Part model, mm, in its own coordinate system. Face numbers are marked on the shaded views. Give positions to 0.01 mm unless a question says otherwise; leave off trailing zeros. Loops run counter-clockwise (first coordinate to the right, second up) from the corner with the lowest first, then second, coordinate; pieces in that order, holes last. Notation, with made-up numbers: (74, 13) -> (133, 13) arc R21 cw to (133, 21) -> close; hole circle Ø2 at (46.5, -21). An arc over 180 degrees is marked (long way). One line per question, with ' | ' between items.
Autodesk Inventor part; units mm, degrees
ref_plane "Work Plane4" through (0, 0, -44.52672) normal (1, 0, 0) x (0, 0.9903099, -0.1388753)
ref_plane "YZ Plane" through (0, 0, 0) normal (1, 0, 0) x (0, 1, 0)
ref_plane "XZ Plane" through (0, 0, 0) normal (0, 1, 0) x (-1, 0, 0)
sketch "Sketch1" plane through (0, 0, 0) normal (0, 1, 0) x (-1, 0, 0)
  circle A0 centre (0, 0) radius 110 construction
  arc A1 (43.0581, -98.5) -> (-43.0581, -98.5) centre (0, 0) ccw
  line L0 (0, -107.5) -> (0, -98.5) construction
  line L1 (0, -98.5) -> (0, -73.5) construction
  line L2 (0, -98.5) -> (-43.0581, -98.5) construction
  line L3 (0, -98.5) -> (43.0581, -98.5) construction
  line L4 (43.0581, -98.5) -> (-43.0581, -98.5) construction
  line L5 (-18.0581, -73.5) -> (18.0581, -73.5)
  arc A2 (43.0581, -98.5) -> (18.0581, -73.5) centre (18.0581, -98.5) ccw
  arc A3 (-18.0581, -73.5) -> (-43.0581, -98.5) centre (-18.0581, -98.5) ccw
  line L6 (0, 107.5) -> (0, 97.5) construction
  line L7 (0, 97.5) -> (-22.5, 97.5) construction
  line L8 (-22.5, 97.5) -> (-22.5, 82.5) construction
  line L9 (22.5, 82.5) -> (22.5, 97.5) construction
  line L10 (22.5, 90) -> (-22.5, 90) construction
  line L11 (15, 97.5) -> (-15, 97.5)
  line L12 (-15, 82.5) -> (15, 82.5)
  arc A4 (15, 82.5) -> (15, 97.5) centre (15, 90) ccw
  arc A5 (-15, 97.5) -> (-15, 82.5) centre (-15, 90) ccw
  line L13 (22.5, 82.5) -> (17.5, 82.5) construction
  line L14 (17.5, 82.5) -> (17.5, 77.5) construction
  circle A6 centre (17.5, 77.5) radius 1.6
  circle A7 centre (-17.5, 77.5) radius 1.6
  line L15 (-58.336309, 79.549513) -> (-79.549513, 58.336309)
  arc A8 (-47.729708, 68.942911) -> (-58.336309, 79.549513) centre (-53.033009, 74.246212) ccw
  arc A9 (-79.549513, 58.336309) -> (-68.942911, 47.729708) centre (-74.246212, 53.033009) ccw
  line L16 (-68.942911, 47.729708) -> (-47.729708, 68.942911)
  circle A10 centre (-67.175144, 42.426407) radius 1.6
  circle A11 centre (-42.426407, 67.175144) radius 1.6
  line L17 (-97.5, 15) -> (-97.5, -15)
  arc A12 (-82.5, 15) -> (-97.5, 15) centre (-90, 15) ccw
  arc A13 (-97.5, -15) -> (-82.5, -15) centre (-90, -15) ccw
  line L18 (-82.5, -15) -> (-82.5, 15)
  circle A14 centre (-77.5, -17.5) radius 1.6
  circle A15 centre (-77.5, 17.5) radius 1.6
  line L19 (-79.549513, -58.336309) -> (-58.336309, -79.549513)
  arc A16 (-68.942911, -47.729708) -> (-79.549513, -58.336309) centre (-74.246212, -53.033009) ccw
  arc A17 (-58.336309, -79.549513) -> (-47.729708, -68.942911) centre (-53.033009, -74.246212) ccw
  line L20 (-47.729708, -68.942911) -> (-68.942911, -47.729708)
  circle A18 centre (-42.426407, -67.175144) radius 1.6
  circle A19 centre (-67.175144, -42.426407) radius 1.6
  line L21 (-15, -97.5) -> (15, -97.5)
  arc A20 (-15, -82.5) -> (-15, -97.5) centre (-15, -90) ccw
  arc A21 (15, -97.5) -> (15, -82.5) centre (15, -90) ccw
  line L22 (15, -82.5) -> (-15, -82.5)
  circle A22 centre (17.5, -77.5) radius 1.6
  circle A23 centre (-17.5, -77.5) radius 1.6
  line L23 (58.336309, -79.549513) -> (79.549513, -58.336309)
  arc A24 (47.729708, -68.942911) -> (58.336309, -79.549513) centre (53.033009, -74.246212) ccw
  arc A25 (79.549513, -58.336309) -> (68.942911, -47.729708) centre (74.246212, -53.033009) ccw
  line L24 (68.942911, -47.729708) -> (47.729708, -68.942911)
  circle A26 centre (67.175144, -42.426407) radius 1.6
  circle A27 centre (42.426407, -67.175144) radius 1.6
  line L25 (97.5, -15) -> (97.5, 15)
  arc A28 (82.5, -15) -> (97.5, -15) centre (90, -15) ccw
  arc A29 (97.5, 15) -> (82.5, 15) centre (90, 15) ccw
  line L26 (82.5, 15) -> (82.5, -15)
  circle A30 centre (77.5, 17.5) radius 1.6
  circle A31 centre (77.5, -17.5) radius 1.6
  line L27 (79.549513, 58.336309) -> (58.336309, 79.549513)
  arc A32 (68.942911, 47.729708) -> (79.549513, 58.336309) centre (74.246212, 53.033009) ccw
  arc A33 (58.336309, 79.549513) -> (47.729708, 68.942911) centre (53.033009, 74.246212) ccw
  line L28 (47.729708, 68.942911) -> (68.942911, 47.729708)
  circle A34 centre (42.426407, 67.175144) radius 1.6
  circle A35 centre (67.175144, 42.426407) radius 1.6
  line L29 (58.336309, -58.336309) -> (51.265242, -51.265242) construction
  line L30 (40.65864, -61.871843) -> (61.871843, -40.65864)
  arc A36 (40.65864, -61.871843) -> (44.52672, -89.539774) centre (53.033009, -74.246212) ccw
  arc A37 (89.539774, -44.52672) -> (61.871843, -40.65864) centre (74.246212, -53.033009) ccw
  line L31 (0, -73.5) -> (0, -66.5) construction
  arc A38 (44.52672, 89.539774) -> (40.65864, 61.871843) centre (53.033009, 74.246212) ccw
  line L32 (61.871843, 40.65864) -> (40.65864, 61.871843)
  arc A39 (61.871843, 40.65864) -> (89.539774, 44.52672) centre (74.246212, 53.033009) ccw
  arc A40 (-89.539774, 44.52672) -> (-61.871843, 40.65864) centre (-74.246212, 53.033009) ccw
  line L33 (-40.65864, 61.871843) -> (-61.871843, 40.65864)
  arc A41 (-40.65864, 61.871843) -> (-44.52672, 89.539774) centre (-53.033009, 74.246212) ccw
  arc A42 (-44.52672, -89.539774) -> (-40.65864, -61.871843) centre (-53.033009, -74.246212) ccw
  line L34 (-61.871843, -40.65864) -> (-40.65864, -61.871843)
  arc A43 (-61.871843, -40.65864) -> (-89.539774, -44.52672) centre (-74.246212, -53.033009) ccw
  arc A44 (89.539774, -44.52672) -> (89.539774, 44.52672) centre (0, 0) ccw
  arc A45 (44.52672, 89.539774) -> (-44.52672, 89.539774) centre (0, 0) ccw
  arc A46 (-89.539774, 44.52672) -> (-89.539774, -44.52672) centre (0, 0) ccw
  line L35 (43.0581, -98.5) -> (48.0581, -98.5) construction
  line L36 (48.0581, -98.5) -> (48.0581, -88.5) construction
  circle A47 centre (48.0581, -88.5) radius 1.6
  circle A48 centre (-48.0581, -88.5) radius 1.6
  line L37 (18.0581, -66.5) -> (-18.0581, -66.5)
  arc A49 (17.5, -66.5) -> (43.0581, -59.472383) centre (19.514525, -23.837671) ccw
  arc A50 (-44.52672, -58.003763) -> (-18.0581, -66.5) centre (-19.508856, -25.542168) ccw
  arc A51 (-48.0581, -88.5) -> (-42.426407, -67.175144) centre (-60.43967, -73.824078) ccw construction
  arc A52 (-48.0581, -88.5) -> (-42.426407, -67.175144) centre (-60.43967, -73.824078) ccw construction
  arc A53 (-44.936716, -92.199789) -> (-37.885276, -65.498953) centre (-60.43967, -73.824078) ccw
  arc A54 (-51.179485, -84.800211) -> (-46.967537, -68.851335) centre (-60.43967, -73.824078) ccw
  arc A55 (-51.179485, -84.800211) -> (-44.936716, -92.199789) centre (-48.0581, -88.5) ccw
  arc A56 (-37.885276, -65.498953) -> (-46.967537, -68.851335) centre (-42.426407, -67.175144) ccw
  line L38 (42.426407, 67.175144) -> (67.175144, 42.426407) construction
  line L39 (45.961941, 70.710678) -> (70.710678, 45.961941)
  line L40 (63.63961, 38.890873) -> (38.890873, 63.63961)
  arc A57 (45.961941, 70.710678) -> (38.890873, 63.63961) centre (42.426407, 67.175144) ccw
  arc A58 (63.63961, 38.890873) -> (70.710678, 45.961941) centre (67.175144, 42.426407) ccw
  line L41 (-42.426407, 67.175144) -> (-67.175144, 42.426407) construction
  line L42 (-45.961941, 70.710678) -> (-70.710678, 45.961941)
  line L43 (-63.63961, 38.890873) -> (-38.890873, 63.63961)
  arc A59 (-38.890873, 63.63961) -> (-45.961941, 70.710678) centre (-42.426407, 67.175144) ccw
  arc A60 (-70.710678, 45.961941) -> (-63.63961, 38.890873) centre (-67.175144, 42.426407) ccw
  line L44 (-42.426407, 67.175144) -> (42.426407, 67.175144) construction
  line L45 (-42.426407, 62.175144) -> (42.426407, 62.175144)
  line L46 (42.426407, 72.175144) -> (-42.426407, 72.175144)
  arc A61 (-42.426407, 72.175144) -> (-42.426407, 62.175144) centre (-42.426407, 67.175144) ccw
  arc A62 (42.426407, 62.175144) -> (42.426407, 72.175144) centre (42.426407, 67.175144) ccw
  line L47 (37.025198, 67.175144) -> (33.025198, 67.175144) construction
  line L48 (33.025198, 67.175144) -> (32.025198, 67.175144) construction
  line L49 (31.025198, 70.425144) -> (31.025198, 63.925144)
  line L50 (31.025198, 63.925144) -> (33.025198, 63.925144)
  line L51 (33.025198, 63.925144) -> (33.025198, 70.425144)
  line L52 (33.025198, 70.425144) -> (31.025198, 70.425144)
  line L53 (31.025198, 70.425144) -> (33.025198, 63.925144) construction
  line L54 (31.025198, 63.925144) -> (33.025198, 70.425144) construction
  line L55 (0, 67.175144) -> (0, 56.50884) construction
  line L56 (-31.025198, 70.425144) -> (-31.025198, 63.925144)
  line L57 (-31.025198, 63.925144) -> (-33.025198, 63.925144)
  line L58 (-33.025198, 63.925144) -> (-33.025198, 70.425144)
  line L59 (-33.025198, 70.425144) -> (-31.025198, 70.425144)
  arc A63 (-43.0581, -98.5) -> (43.0581, -98.5) centre (0, 0) ccw
  line L60 (0, -107.5) -> (0, -103.5)
  arc A64 (-41.455938, -94.834884) -> (41.455938, -94.834884) centre (0, 0) ccw
  arc A65 (41.455938, -94.834884) -> (42.699608, -94.281459) centre (0, 0) ccw
  arc A66 (-42.699608, -94.281459) -> (-41.455938, -94.834884) centre (0.000004, 0.000008) ccw
  point P0 (0, 90)
  point P1 (-45.961941, 70.710678)
  point P2 (-82.5, 17.5)
  point P3 (-70.710678, -45.961941)
  point P4 (-17.5, -82.5)
  point P5 (45.961941, -70.710678)
  point P6 (82.5, -17.5)
  point P7 (70.710678, 45.961941)
  point P8 (35.715922, -76.769806)
  point P9 (-37.90233, -65.453455)
  point P10 (-39.097126, -63.661261)
  point P11 (-46.422064, -70.704261)
  point P12 (-46.867306, -78.516354)
  point P13 (0, -44.52672)
  point P14 (0, 35.701561)
  point P15 (54.800776, 54.800776)
  point P16 (-54.800776, 54.800776)
  point P17 (40.355339, 62.175144)
  point P18 (40.65864, 61.871843)
  point P19 (-47.729708, 68.942911)
  point P20 (-68.942911, 47.729708)
  point P21 (-61.871843, 40.65864)
  point P22 (-40.355339, 62.175144)
  dimension "d0" = 220
  dimension "d1" = 215
  dimension "d2" = 9
  dimension "d3" = 25
  dimension "d4" = 10
  dimension "d5" = 22.5
  dimension "d6" = 15
  dimension "d7" = 45
  dimension "d8" = 5
  dimension "d9" = 5
  dimension "d10" = 3.2
  dimension "d15" = 86.1162
  dimension "d16" = 45
  dimension "d19" = 360
  dimension "d22" = 10
  dimension "d23" = 7
  dimension "d26" = 360
  dimension "d33" = 5
  dimension "d34" = 10
  dimension "d35" = 3.2
  dimension "d68" = 4
  dimension "d69" = 1
  dimension "d70" = 6.5
  dimension "d71" = 2
  dimension "d123" = 4
ref_plane "Work Plane4" through (0, 0, -44.52672) normal (1, 0, 0) x (0, 0.9903099, -0.1388753)
extrude "Extrusion13" add sketch "Sketch1" against normal blind 30 contours A63 L60 A64 A65 A2 | A3 A66 A64 L60 A63
properties part number "MettalringUnten_v3"
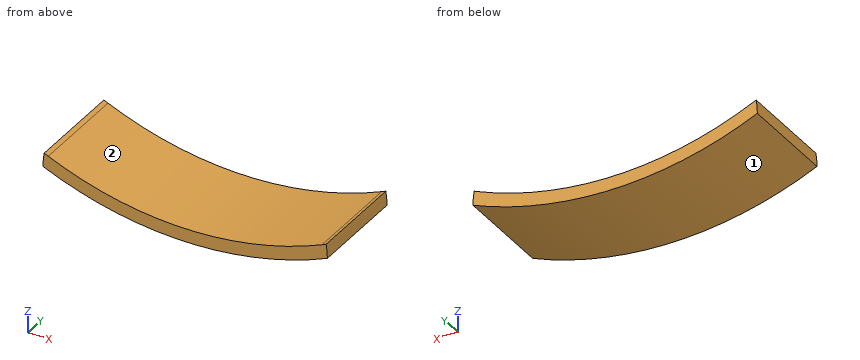
1) Drill centre lines: line 1 (Z direction, x = -1, y = -20.5); line 2 (Z direction, x = -27, y = -3.25). Where is each one in solid material? Low to high.
Found:
line 1: -107.5 to -103.5 | line 2: -104.05 to -99.92
2) Pin check, flat tips, straight feed: P1, Ø10, axis at x = -26, y = -22.5, coming from the +Z side; P2, Ø8, axis at x = 24, y = -25, coming from the +Z side; P3, Ø1.5, axis at y = -7.5, z = -96.5, coming from the +X side. Stop position of each tip, or through.
Found:
P1: z = -98.75 | P2: z = -99.64 | P3: x = 43.03
3) Saw through at C-C (z = -96.75). Give the cut face in (x, y).
Found:
outline: (-43, -30) -> (-36.77, -30) -> (-36.77, 0) -> (-43, 0) -> close; (36.77, -30) -> (43, -30) -> (43, 0) -> (36.77, 0) -> close
4) Saw through at B-B (y = -26.75). Give the cut face in (x, z), and give its area (3 significant figures).
Found:
outline: (-43.06, -98.5) arc R107.5 ccw to (43.06, -98.5) arc R25 ccw to (42.7, -94.28) arc R103.5 cw to (41.46, -94.83) arc R103.5 cw to (-41.46, -94.83) arc R103.5 cw to (-42.7, -94.28) arc R25 ccw to start | area: 354 mm2
5) Pull direction X, two halves, no side cores. Call the marked faces 1 and 2: pulls with the +X half, pulls with the -X half, needs draft (parallel to the pull), parting line crosses it, or undercut.
Found:
face 1: parting line crosses it | face 2: undercut
6) Saw through at D-D (x = 17). Give the cut face in (y, z), and give its area (3 significant figures).
Found:
outline: (-30, -106.15) -> (0, -106.15) -> (0, -102.09) -> (-30, -102.09) -> close | area: 122 mm2
7) Saw through at A-A (z = -100.5). Give the cut face in (x, y).
Found:
outline: (-38.16, -30) -> (-24.74, -30) -> (-24.74, 0) -> (-38.16, 0) -> close; (24.74, -30) -> (38.16, -30) -> (38.16, 0) -> (24.74, 0) -> close
